For this review, take the finished solid that the model builds, in its own axes (mm). A direction names the side the tool comes from. Round coordinates to 2 decimals unless told otherwise and drop trailing zeros. Loops run counter-clockwise (first coordinate to the right, second up) from the corner with the lowest first, then second, coordinate; pieces in that order, holes last.
1. Clearance check with flat-ended pins moving along their axes: pin 1 Ø12 at (x, z) = (7, 14.5) entering from -Y; pin 2 Ø4 at (x, y) = (18, 5.5) entering from +Z. State where each tip first meets the part, or that it passes through.
2. Consider section A-A on z = 7.5. State the section outline as (x, y) points.
3. To check wall thickness, follow line 1 along X through (y, z) = (6, 11.25); line 2 along Z through (x, y) = (5, 9.5); line 3 along Y through (x, z) = (21, 15.75). State the ranges of each line that lie inside material, in increasing order.
4. Consider section D-D on z = 18. State the section outline as (x, y) points.
5. Draft analysis for pull direction Y (two halves, no side actions). For faces 5 (the flat face through (7, 6, 17.5)), 6 (the cylindrical face through (23.255, 6.706, 11.162)), 7 (the flat face through (12, 0, 10)), 8 (the cylindrical face through (16.865, 6.025, -1.268)), state which applies: released by +Y, released by -Y, zero draft, split by the parting line, or undercut.
6. Consider section B-B on z = -1. State the section outline as (x, y) points, then the cut area to 3 significant figures.
7. Consider section C-C on x = 22.66. State the section outline as (y, z) points.
8. Tool access review of faces 1 (the cylindrical face through (23.255, 6.706, -1.268)), 2 (the flat face through (12, 2.5, 12)), 3 (the cylindrical face through (3.09, 6.22, 11.16)), 4 (the flat face through (18, 6, 17.5)): name each direction out of +Z, -Z, +X, -X, +Y, -Y from which nothing blocks a thin tool from reaching the whole face with its end or side.
from build123d import *

# Parameters (mm, degrees)
SKETCH_1_W           = 25
SKETCH_1_H           = 10
EXTRUDE_1_DEPTH      = 5
SKETCH_2_W           = 25
SKETCH_2_H           = 2.5
EXTRUDE_2_DEPTH      = 15
EXTRUDE_3_DEPTH      = 12.5
EXTRUDE_3_DEPTH_BACK = 7.5
SKETCH_3_R           = 0.75


with BuildPart() as part:
    # Sketch 1 → Extrude 1 (new body)
    with BuildSketch(Plane.XY):
        with Locations((12.5, 5)):
            Rectangle(SKETCH_1_W, SKETCH_1_H)
    extrude(amount=EXTRUDE_1_DEPTH)

    # Sketch 2 → Extrude 2 (add)
    with BuildSketch(Plane.XY.offset(5)):
        with Locations((12.5, 1.25)):
            Rectangle(SKETCH_2_W, SKETCH_2_H)
    extrude(amount=EXTRUDE_2_DEPTH)

    # Sketch 3 → Extrude 3 (add, two sides: drawn at the far end of the back side and taken through both)
    with BuildSketch(Plane.XY.offset(5).offset(-EXTRUDE_3_DEPTH_BACK)):
        with Locations(Location((17.58, 6.25, 0), (0, 0, 180))):
            Circle(SKETCH_3_R)
        with Locations(Location((22.66, 6.25, 0), (0, 0, 180))):
            Circle(SKETCH_3_R)
        with Locations(Location((2.34, 6.25, 0), (0, 0, 180))):
            Circle(SKETCH_3_R)
        with Locations(Location((7.42, 6.25, 0), (0, 0, 180))):
            Circle(SKETCH_3_R)
        with Locations(Location((12.5, 6.25, 0), (0, 0, 180))):
            Circle(SKETCH_3_R)
    extrude(amount=EXTRUDE_3_DEPTH + EXTRUDE_3_DEPTH_BACK)


solid = part.part
Resolved:
1. pin 1: stops at y = 0
1. pin 2: stops at z = 17.5
2. outline: (0, 0) - (25, 0) - (25, 2.5) - (0, 2.5) - close; circle Ø1.5 at (2.34, 6.25); circle Ø1.5 at (7.42, 6.25); circle Ø1.5 at (12.5, 6.25); circle Ø1.5 at (17.58, 6.25); circle Ø1.5 at (22.66, 6.25)
3. line 1: x = 1.63 to 3.05, 6.71 to 8.13, 11.79 to 13.21, 16.87 to 18.29, 21.95 to 23.37
3. line 2: z = 0 to 5
3. line 3: y = 0 to 2.5
4. outline: (0, 0) - (25, 0) - (25, 2.5) - (0, 2.5) - close
5. face 5: zero draft
5. face 6: undercut
5. face 7: released by -Y
5. face 8: split by the parting line
6. outline: circle Ø1.5 at (2.34, 6.25); circle Ø1.5 at (7.42, 6.25); circle Ø1.5 at (12.5, 6.25); circle Ø1.5 at (17.58, 6.25); circle Ø1.5 at (22.66, 6.25)
6. area: 8.84 mm2
7. outline: (0, 0) - (5.5, 0) - (5.5, -2.5) - (7, -2.5) - (7, 0) - (10, 0) - (10, 5) - (7, 5) - (7, 17.5) - (5.5, 17.5) - (5.5, 5) - (2.5, 5) - (2.5, 20) - (0, 20) - close
8. face 1: -Z
8. face 2: +Z, +X, -X
8. face 3: +Z
8. face 4: +Z, +X, -X, +Y
